Verification items for the finished model (mm, model axes). Face numbers are marked on the shaded views. Coordinates: 2 decimals unless noted, no trailing zeros. Order: outer loops, then holes, each group sorted by start corner. A loop starts at its lowest first (then second) coordinate and runs counter-clockwise, first axis right, second up. Notation, with made-up numbers: M -16.5,44.25 L 19.5,44.25 A33 ccw 19.5,79.25 Z; hole C 12.5,-23 d8. An arc over 180 degrees is marked long. Return JSON: item names as keys, results as strings.
```python
from build123d import *

# Parameters (mm, degrees)
F0_W         = 101.6
F0_H         = 76.2
F1_DEPTH     = 152.4
F2_T         = -7.62
F3_R         = 39.7017420332
F1_FACE_W    = 76.2
F1_FACE_H    = 152.4
F5_T3_ANGLE  = 90
F5_T6_DEPTH  = 21.2582579668
F5_T9_DEPTH  = 46.6582579668
F5_S10_R     = 152.4
F5_T11_DEPTH = 25


# Not quite as in the source:
# - a fillet or chamfer that OpenCascade refuses, or shapes differently, is made with other operations: its cross-section is extruded or revolved along the edge and cut away or added


with BuildPart() as f1:
    # F0 (on Top) → F1 (new body)
    with BuildSketch(Plane.XY):
        with Locations((-6.3440203667, 13.8422726145)):
            Rectangle(F0_W, F0_H)
    extrude(amount=F1_DEPTH)

    # F2
    f2_openings = [f1.faces().sort_by_distance(p)[0] for p in [
        (-6.34402, 13.842273, 152.4),
    ]]
    offset(amount=F2_T, openings=f2_openings)

    # F3
    f3_edges = [f1.edges().sort_by_distance(p)[0] for p in [
        (-49.52402, -16.637727, 80.01),
    ]]
    fillet(f3_edges, radius=F3_R)

    # F1_face (on face) → F4 (revolve)
    with BuildSketch(Plane(origin=(44.4559796333, 13.8422726145, 76.2), x_dir=(0, 1, 0), z_dir=(1, 0, 0))):
        Rectangle(F1_FACE_W, F1_FACE_H)
    revolve(axis=Axis((44.4559796333, 13.8422726145, 0), (0, -1, 0)))

    # F5: fillet of radius 0.2414213562 on 1 edges, made by hand


with BuildPart() as f5_tool1:
    # F5_s2 → F5_t3 (revolve)
    with BuildSketch(Plane.XZ.offset(-23.0640146477)):
        with BuildLine():
            ThreePointArc((-49.7654417229, 152.4), (-49.5947310448, 152.3292893219), (-49.5240203667, 152.1585786438))
            Line((-49.5240203667, 152.1585786438), (-49.5240203667, 152.4))
            Line((-49.5240203667, 152.4), (-49.7654417229, 152.4))
        make_face()
    revolve(axis=Axis((-9.8222783334, 23.0640146477, 152.4), (0, 0, 1)), revolution_arc=F5_T3_ANGLE)


with BuildPart() as f5_tool4:
    # F5_s5 → F5_t6 (new body)
    with BuildSketch(Plane.XZ.offset(-44.3222726145)):
        with BuildLine():
            ThreePointArc((-49.7654417229, 152.4), (-49.5947310448, 152.3292893219), (-49.5240203667, 152.1585786438))
            Line((-49.5240203667, 152.1585786438), (-49.5240203667, 152.4))
            Line((-49.5240203667, 152.4), (-49.7654417229, 152.4))
        make_face()
    extrude(amount=F5_T6_DEPTH)


with BuildPart() as f5_tool7:
    # F5_s8 → F5_t9 (new body)
    with BuildSketch(Plane.YZ.offset(-9.8222783334)):
        with BuildLine():
            ThreePointArc((-16.8791487417, 152.4), (-16.7084380636, 152.3292893219), (-16.6377273855, 152.1585786438))
            Line((-16.6377273855, 152.1585786438), (-16.6377273855, 152.4))
            Line((-16.6377273855, 152.4), (-16.8791487417, 152.4))
        make_face()
    extrude(amount=F5_T9_DEPTH)

    # F5_s10 → F5_t11 (cut, symmetric)
    with BuildSketch(Plane.XZ.offset(16.8)):
        with Locations((44.4559796333, 0)):
            Circle(F5_S10_R)
    extrude(amount=F5_T11_DEPTH, both=True, mode=Mode.SUBTRACT)


with BuildPart() as f1_1:
    add(f1.part)

    # F5_t12: cut F5_tool1, F5_tool4, F5_tool7
    add([f5_tool1.part, f5_tool4.part, f5_tool7.part], mode=Mode.SUBTRACT)


solid = f1_1.part
```
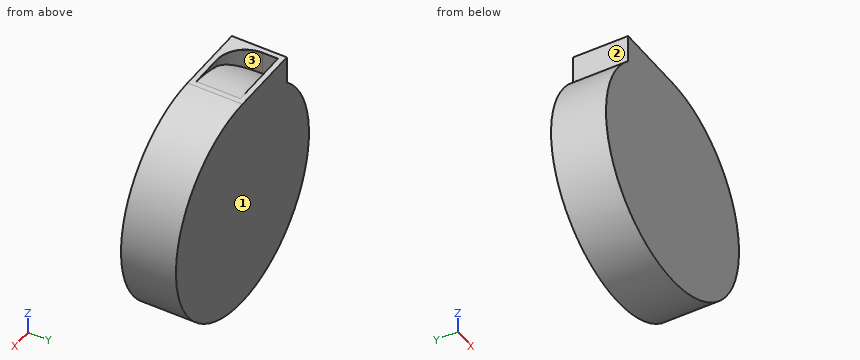
Q1. Cross-section at A-A, the plane y = 35. Record the boundary of the cut face in (x, z).
Values:
{"outline": "M -57.14,113.59 A152.4 ccw long 44.46,152.4 L 36.84,152.4 L 36.84,152.21 A152.4 ccw -49.52,119.97 L -49.52,152.16 A0.24 ccw -49.77,152.4 L -57.14,152.4 Z"}
Q2. Cross-section at D-D, the plane z = -77. Record the boundary of the cut face in (x, y).
Values:
{"outline": "M -87.06,-24.26 L 175.97,-24.26 L 175.97,51.94 L -87.06,51.94 Z"}
Q3. Go/stop test with flat-tipped pins: pin 1 (5 mm diameter, centred on x = 150, y = -12, fed in from -Z); pin 2 (1 mm diameter, centred on y = 19.5, z = -108.5, fed in from -X); pin 3 (10.5 mm diameter, centred on y = 36.5, z = 133, fed in from +X). Record where each tip stops, or that it passes through.
Values:
{"pin 1": "z = -112.28", "pin 2": "x = -63.07", "pin 3": "x = 127.56"}
Q4. Cross-section at B-B, the plane z = 125. Record the boundary of the cut face in (x, y), and give its area (3 significant figures).
Values:
{"outline": "M -57.14,-24.26 L 131.64,-24.26 L 131.64,51.94 L -57.14,51.94 Z; hole M -49.52,23.06 A39.7 ccw -42.73,0.85 L -42.73,44.32 L -49.52,44.32 Z", "area": "14,100 mm^2"}
Q5. Draft check along Y on the marked faces 1, 2 and 3. Enter one of: pulls with the +Y half, pulls with the -Y half, needs draft (parallel to the pull), parting line crosses it, or undercut.
Values:
{"face 1": "pulls with the +Y half", "face 2": "needs draft", "face 3": "undercut"}
Q6. Cross-section at C-C, the plane z = 85. Record the boundary of the cut face in (x, y).
Values:
{"outline": "M -82.04,-24.26 L 170.95,-24.26 L 170.95,51.94 L -82.04,51.94 Z"}
Q7. Material ranges on line 1 along Z through (x, y) = (49, 40.5); line 2 along X through (y, z) = (39.5, 131); line 3 along Z through (x, y) = (117.5, 10), recorded low to high.
Values:
{"line 1": "-152.33 to 152.33", "line 2": "-57.14 to -49.52, -33.42 to 122.33", "line 3": "-133.75 to 133.75"}
